```python
from build123d import *

# Parameters (mm, degrees)
ESTRUSIONE_ESTRUSIONE1_DEPTH = 3
RACCORDO1_R                  = 10
SCHIZZO2_R                   = 1.75
TAGLIO_ESTRUSIONE1_DEPTH     = 3
SMUSSO1_SIZE                 = 1.5
SCHIZZO4_R                   = 1.75
SCHIZZO4_R_2                 = 1.5
TAGLIO_ESTRUSIONE2_DEPTH     = 230.558271469
SCHIZZO3_R                   = 1.75
TAGLIO_ESTRUSIONE3_DEPTH     = 10
SMUSSO2_SIZE                 = 1.5


with BuildPart() as part:
    # Schizzo1 → Estrusione-Estrusione1 (new body)
    with BuildSketch(Plane.XY):
        Polygon((172, 152), (55.74011537, 152), (-2, 94.25988463), (-2, -2), (172, -2), align=None)
    extrude(amount=ESTRUSIONE_ESTRUSIONE1_DEPTH)

    # Raccordo1
    raccordo1_edges = [part.edges().sort_by_distance(p)[0] for p in [
        (172, -2, 1.5),
        (-2, -2, 1.5),
        (-2, 94.25988463, 1.5),
        (55.74011537, 152, 1.5),
        (172, 152, 1.5),
    ]]
    fillet(raccordo1_edges, radius=RACCORDO1_R)

    # Schizzo2 → Taglio-Estrusione1 (cut)
    with BuildSketch(Plane.XY.offset(3)):
        with Locations((162, 142)):
            Circle(SCHIZZO2_R)
        with Locations((59.882250994, 142)):
            Circle(SCHIZZO2_R)
        with Locations((8, 90.117749006)):
            Circle(SCHIZZO2_R)
        with Locations((8, 8)):
            Circle(SCHIZZO2_R)
        with Locations((162, 8)):
            Circle(SCHIZZO2_R)
        with Locations((162, 73.82941029)):
            Circle(SCHIZZO2_R)
        with Locations((83.881838923, 8)):
            Circle(SCHIZZO2_R)
    extrude(amount=-TAGLIO_ESTRUSIONE1_DEPTH, mode=Mode.SUBTRACT)

    # Smusso1
    smusso1_edges = [part.edges().sort_by_distance(p)[0] for p in [
        (58.132250994, 142, 3),
        (6.25, 90.117749006, 3),
        (6.25, 8, 3),
        (160.25, 8, 3),
        (160.25, 73.82941029, 3),
        (82.131838923, 8, 3),
        (160.25, 142, 3),
    ]]
    chamfer(smusso1_edges, length=SMUSSO1_SIZE)

    # Schizzo4 → Taglio-Estrusione2 (cut, through all)
    with BuildSketch(Plane.XY.offset(3)):
        with Locations((150.4, 97)):
            Circle(SCHIZZO4_R)
        with Locations((142, 83)):
            Circle(SCHIZZO4_R)
        with Locations((79.8, 83)):
            Circle(SCHIZZO4_R)
        with Locations((152, 79.499997822)):
            Circle(SCHIZZO4_R_2)
    extrude(amount=-TAGLIO_ESTRUSIONE2_DEPTH, mode=Mode.SUBTRACT)

    # Schizzo3 → Taglio-Estrusione3 (cut)
    with BuildSketch(Plane(origin=(0, 0, 0), x_dir=(-1, 0, 0), z_dir=(0, 0, -1))):
        with Locations((-61.6, 79)):
            Circle(SCHIZZO3_R)
        with Locations((-6.6, 79)):
            Circle(SCHIZZO3_R)
        with Locations((-6.6, 19)):
            Circle(SCHIZZO3_R)
        with Locations((-61.6, 19)):
            Circle(SCHIZZO3_R)
    extrude(amount=-TAGLIO_ESTRUSIONE3_DEPTH, mode=Mode.SUBTRACT)

    # Smusso2
    smusso2_edges = [part.edges().sort_by_distance(p)[0] for p in [
        (148.65, 97, 0),
        (140.25, 83, 0),
        (78.05, 83, 0),
        (63.35, 19, 3),
        (8.35, 19, 3),
        (8.35, 79, 3),
        (63.35, 79, 3),
    ]]
    chamfer(smusso2_edges, length=SMUSSO2_SIZE)


solid = part.part
```
The listing builds one solid part. Answer for the finished solid, in the listing's coordinates (mm). Round coordinates to 2 decimals unless told otherwise and drop trailing zeros. Order: outer loops, then holes, each group sorted by start corner. A loop starts at its lowest first (then second) coordinate and runs counter-clockwise, first axis right, second up. Notation, with made-up numbers: (-15, 67) - (24, 67) arc R13 cw to (24, 92) - close; hole circle Ø6 at (-39, 51.5). An arc over 180 degrees is marked (long way). Put each result on its own line as item: value. Start each with the question number.
(1) Find section B-B (x = 34.5). Give the vertices of the cut face in (y, z).
(2) Given P1, Ø4.5, axis at x = 150.4, y = 97, coming from the -Z side; P2, Ø5.5, axis at x = 8, y = 90.12, coming from the +Z side; P3, Ø4, axis at x = 142, y = 83, coming from the -Z side, each flat-ended and moving along its own axis, determine where each tip first touches the part or whether it passes through.
(3) Determine the mould class of faces 1 (the cylindrical face through (168.99, 0.85, 1.52)), 2 (the cylindrical face through (7.62, 88.41, 0.76)), 3 (the cylindrical face through (168.99, 149.15, 1.52)), 4 (the flat face through (84, 76, 3)) for opening direction Y: released by +Y, released by -Y, zero draft, split by the parting line, or undercut.
(4) Straight lines are drawn through the part: probe 1 along Y at (x, z) = (162, 1.1); probe 2 along X at (y, z) = (83, 2.35); probe 3 along Y at (x, z) = (79.8, 2.5). For each, find the intervals that lie inside material, in ascending order. Write a range as from..to.
(5) Find section A-A (z = 2.5). State how many separate pieces and enclosed holes the cut face has, plus the area to 3 significant figures.
Reply:
1. outline: (-2, 0) - (130.76, 0) - (130.76, 3) - (-2, 3) - close
2. P1: z = 1
2. P2: z = 2.5
2. P3: z = 1.25
3. face 1: released by -Y
3. face 2: undercut
3. face 3: released by +Y
3. face 4: zero draft
4. probe 1: -2..6.25, 9.75..72.08, 75.58..140.25, 143.75..152
4. probe 2: -2..78.05, 81.55..140.25, 143.75..172
4. probe 3: -2..81.25, 84.75..152
5. separate pieces: 1
5. enclosed holes: 15
5. area: 24,800 mm^2
